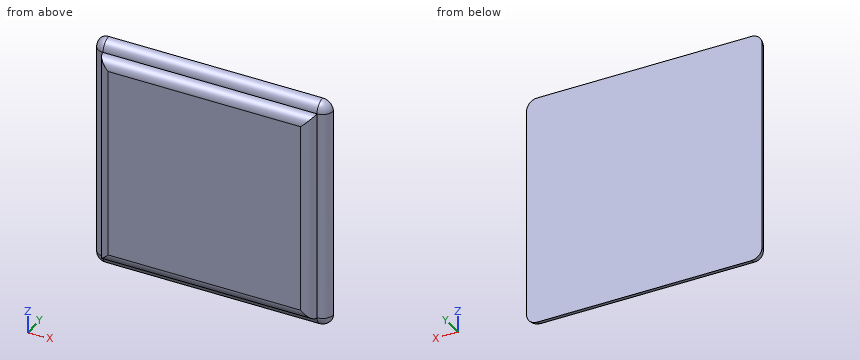
from build123d import *

# Parameters (mm, degrees)
F0_W     = 100
F0_H     = 100
F1_DEPTH = 5
F2_W     = 110
F2_H     = 110
F3_DEPTH = 5
F4_R     = 5
F5_R     = 4.99999
F6_R     = 4.99999


# Not quite as in the source:
# - a fillet or chamfer is up to 0.001 mm smaller than in the source, because OpenCascade refuses the exact size


with BuildPart() as f1:
    # F0 (on Front) → F1 (new body)
    with BuildSketch(Plane.XZ):
        Rectangle(F0_W, F0_H)
    extrude(amount=F1_DEPTH)

    # F2 (on face) → F3 (join)
    with BuildSketch(Plane(origin=(0, 0, 0), x_dir=(-1, 0, 0), z_dir=(0, 1, 0))):
        Rectangle(F2_W, F2_H)
    extrude(amount=F3_DEPTH)

    # F4
    f4_edges = [f1.edges().sort_by_distance(p)[0] for p in [
        (-55, 2.5, -55),
        (55, 2.5, -55),
        (55, 2.5, 55),
        (-55, 2.5, 55),
    ]]
    fillet(f4_edges, radius=F4_R)

    # F5 (radius 5 in the source; OpenCascade refuses exactly that, so slightly less here)
    f5_edges = [f1.edges().sort_by_distance(p)[0] for p in [
        (0, -5, 50),
        (50, -5, 0),
        (0, -5, -50),
        (-50, -5, 0),
    ]]
    fillet(f5_edges, radius=F5_R)

    # F6 (radius 5 in the source; OpenCascade refuses exactly that, so slightly less here)
    f6_edges = [f1.edges().sort_by_distance(p)[0] for p in [
        (0, 0, -55),
    ]]
    fillet(f6_edges, radius=F6_R)


solid = f1.part
Source: CAD feature listing. Evaluate the final solid. Frame: model axes, mm. Round coordinates to 2 decimals unless told otherwise and drop trailing zeros. Loops run counter-clockwise (first coordinate to the right, second up) from the corner with the lowest first, then second, coordinate; pieces in that order, holes last. Notation, with made-up numbers: M 59.5,24 L 90.5,24 A23 cw 90.5,37 Z; hole C 72.25,24 d10. An arc over 180 degrees is marked long. Answer as CSV lines item,"result".
Q1. Cut plane C-C (y = -3). Return the cut outline in (x, z).
Verdict:
outline,"M -49,-49 L 49,-49 L 49,49 L -49,49 Z"
Q2. Contact query for flat-ended pins moving along their axis: pin 1 (5 mm diameter, centred on x = -35.5, y = 1, fed in from +Z); pin 2 (1 mm diameter, centred on x = -34.5, y = 2.5, fed in from +Z); pin 3 (2 mm diameter, centred on x = 7, y = 0.5, fed in from -Z). Output: stop coordinate, or through.
Verdict:
pin 1,"stops at z = 54.77"
pin 2,"stops at z = 54.58"
pin 3,"stops at z = -53.57"
Q3. Line query: line 1 along X through (y, z) = (-0.5, 25.5); line 2 along Y through (x, z) = (-45.5, 30); line 3 along X through (y, z) = (4.5, -36). Output: solid intervals per line, ascending.
Verdict:
line 1,"x = -49.97 to 49.97"
line 2,"y = -4.97 to 5"
line 3,"x = -54.97 to 54.97"
